Part print with two shaded views. Sizes in mm from the minimum x, y, z corner. A direction names the side the tool comes from. Round coordinates to 2 decimals unless told otherwise and drop trailing zeros. Write each loop counter-clockwise with the first axis right and the second up, starting at its lowest first coordinate (ties: lowest second). Pieces come first, ordered by that corner, then holes. Notation, with made-up numbers: (14.5, 86.5) - (63.5, 86.5) arc R23 ccw to (63.5, 125.5) - close; hole circle Ø3 at (35, 34.25). An arc over 180 degrees is marked (long way). Use one line per item in the form item = value. Start each with the question number.
Item 1: Pin check, flat tips, straight feed: pin 1 (3 mm diameter, centred on y = 72.5, z = 7.5, fed in from +X); pin 2 (1 mm diameter, centred on x = 18, y = 28.5, fed in from +Z); pin 3 (3 mm diameter, centred on y = 87, z = 20.5, fed in from -X). Stop position of each tip, or through.
Item 2: Band-saw the part on A-A, the plane z = 16. List the corners of the cut face in (x, y).
Item 3: Band-saw the part on D-D, the plane y = 77. List the corners of the cut face in (x, z), and give its area (3 significant figures).
Item 4: Drill centre lines: L1, parallel to Y at x = 23, z = 6.5; L2, parallel to Y at x = 27, z = 20.5; L3, parallel to X at y = 48.5, z = 9. Where is each one in solid material? Low to high.
Item 5: Tool access for the marked faces 5, 6, 7, 8 and 9: list every direction of +Z, -Z, +X, -X, +Y, -Y with a clear straight run to the whole face (end or side of a thin tool).
Item 6: Pull direction Y, two halves, no side cores. Call the marked faces 1, 2, 3 and 4: +Y half, -Y half, draft (parallel to the pull), parting line (faces both ways), or undercut.
Item 7: Band-saw the part on C-C, the plane y = 52.5. List the corners of the cut face in (x, z), and give its area (3 significant figures).
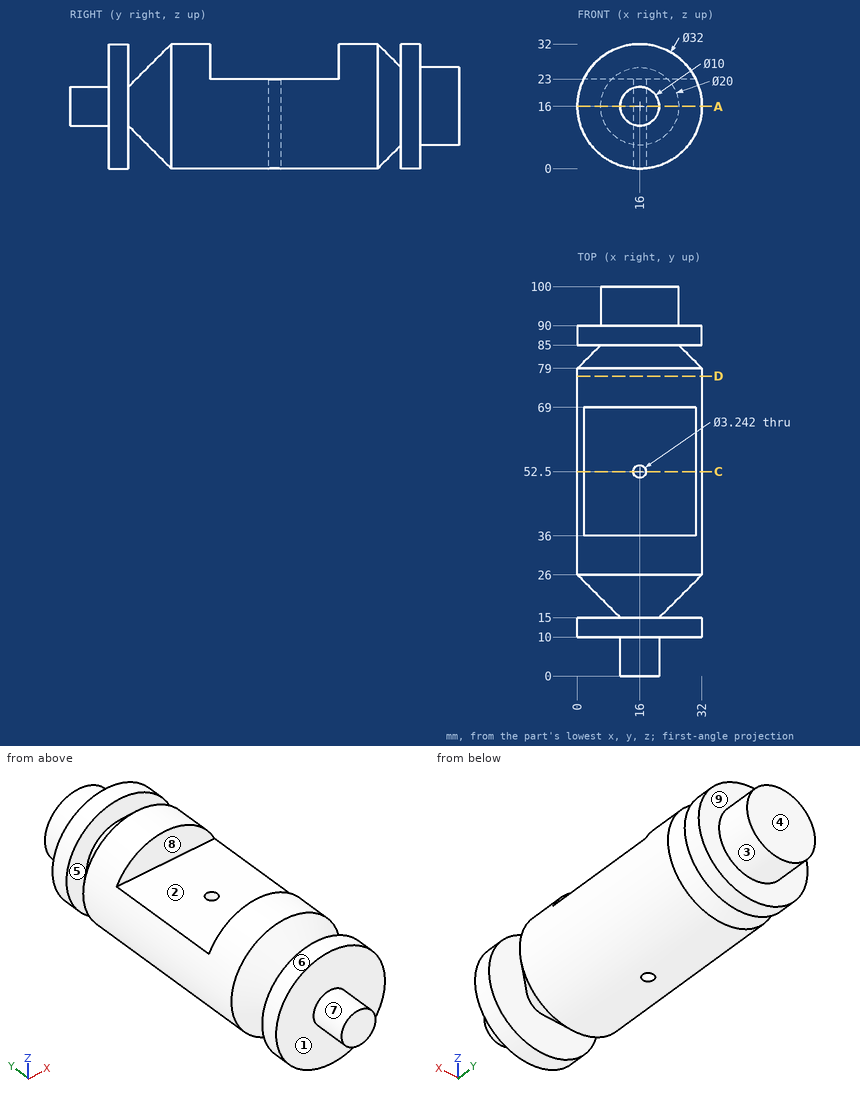
Determined:
q1.pin_1 = 30.39
q1.pin_2 = 31.93
q1.pin_3 = 0.28
q2.outline = (0, 10) - (11, 10) - (11, 0) - (21, 0) - (21, 10) - (32, 10) - (32, 15) - (21, 15) - (32, 26) - (32, 79) - (26, 85) - (32, 85) - (32, 90) - (26, 90) - (26, 100) - (6, 100) - (6, 90) - (0, 90) - (0, 85) - (6, 85) - (0, 79) - (0, 26) - (11, 15) - (0, 15) - close; hole circle Ø3.24 at (16, 52.5)
q3.outline = circle Ø32 at (16, 16)
q3.area = 804 mm²
q4.L1 = 10 to 15, 21.8 to 83.2, 85 to 90
q4.L2 = 10 to 15, 21.88 to 83.12, 85 to 90
q4.L3 = 1.61 to 30.39
q5.face_5 = none
q5.face_6 = +Y, -Y
q5.face_7 = -Y
q5.face_8 = +Z, +X, -X
q5.face_9 = +Y
q6.face_1 = -Y half
q6.face_2 = undercut
q6.face_3 = draft
q6.face_4 = +Y half
q7.outline = (1.61, 23) arc R16 ccw to (14.38, 0.08) - (14.38, 23) - close; (17.62, 0.08) arc R16 ccw to (30.39, 23) - (17.62, 23) - close
q7.area = 544 mm²
